Verification items for the finished model (mm, model axes). A direction names the side the tool comes from. Round coordinates to 2 decimals unless told otherwise and drop trailing zeros. Write each loop counter-clockwise with the first axis right and the second up, starting at its lowest first coordinate (ties: lowest second). Pieces come first, ordered by that corner, then holes.
from build123d import *

# Parameters (mm, degrees)
CYLINDER002_R          = 7
CYLINDER002_DEPTH      = 15
CYLINDER002_ROLL_ANGLE = -90
PAD_DEPTH              = 15
CYLINDER003_R          = 12
CYLINDER003_DEPTH      = 30
CYLINDER_R             = 11
CYLINDER_DEPTH         = 7
BOX_W                  = 30
BOX_H                  = 15
BOX_DEPTH              = 30
CYLINDER001_R          = 15
CYLINDER001_DEPTH      = 15
CYLINDER001_ROLL_ANGLE = -90
CYLINDER004_R          = 15
CYLINDER004_DEPTH      = 45


with BuildPart() as cylinder001:
    # Cylinder002 → Cylinder002 (new body)
    with BuildSketch(Plane.XY):
        Circle(CYLINDER002_R)
    extrude(amount=CYLINDER002_DEPTH)


with BuildPart() as cylinder001_1:
    # Cylinder002 roll: moved
    add(cylinder001.part.rotate(Axis((0, 0, 0), (1, 0, 0)), CYLINDER002_ROLL_ANGLE))


with BuildPart() as cylinder001_2:
    # Cylinder002 placement: moved
    add(cylinder001_1.part.moved(Location((0, -7.5, 0))))


with BuildPart() as body:
    # Sketch → Pad (new body)
    with BuildSketch(Plane.XZ):
        Polygon((-7, 0), (7, 0), (15, -8), (15, -30), (-15, -30), (-15, -8), align=None)
    extrude(amount=-PAD_DEPTH)


with BuildPart() as body_1:
    # Body placement: moved
    add(body.part.moved(Location((0, -7.5, 0))))


with BuildPart() as common:
    # Cylinder003 → Cylinder003 (new body)
    with BuildSketch(Plane.XY.offset(-30)):
        Circle(CYLINDER003_R)
    extrude(amount=CYLINDER003_DEPTH)

    # Common: intersect Body
    add(body_1.part, mode=Mode.INTERSECT)


with BuildPart() as negative_fusion:
    # Cylinder → Cylinder (new body)
    with BuildSketch(Plane(origin=(0, -3.5, 0), x_dir=(0, 0, -1), z_dir=(0, 1, 0))):
        Circle(CYLINDER_R)
    extrude(amount=CYLINDER_DEPTH)

    # Fusion: union Cylinder001, Common
    add(cylinder001_2.part)
    add(common.part)


with BuildPart() as cube:
    # Box → Box (new body)
    with BuildSketch(Plane(origin=(-15, -7.5, -30), x_dir=(1, 0, 0), z_dir=(0, 0, 1))):
        with Locations((15, 7.5)):
            Rectangle(BOX_W, BOX_H)
    extrude(amount=BOX_DEPTH)


with BuildPart() as cut:
    # Cylinder001 → Cylinder001 (new body)
    with BuildSketch(Plane.XY):
        Circle(CYLINDER001_R)
    extrude(amount=CYLINDER001_DEPTH)


with BuildPart() as cut_1:
    # Cylinder001 roll: moved
    add(cut.part.rotate(Axis((0, 0, 0), (1, 0, 0)), CYLINDER001_ROLL_ANGLE))


with BuildPart() as cut_2:
    # Cylinder001 placement: moved
    add(cut_1.part.moved(Location((0, -7.5, 0))))

    # Fusion001: union Cube
    add(cube.part)

    # Cut: cut Negative Fusion
    add(negative_fusion.part, mode=Mode.SUBTRACT)


with BuildPart() as common001:
    # Cylinder004 → Cylinder004 (new body)
    with BuildSketch(Plane.XY.offset(-30)):
        Circle(CYLINDER004_R)
    extrude(amount=CYLINDER004_DEPTH)

    # Common001: intersect Cut
    add(cut_2.part, mode=Mode.INTERSECT)


solid = common001.part
Q1. Sectioned sample at C-C (y = -0.75). Enter the section's corners in (x, z), plus the area to 3 significant figures.
Recorded:
outline: (-14.98, -30) - (-11.98, -30) - (-11.98, -4.98) - (-10.45, -3.45) arc R11 cw (long way) to (10.45, -3.45) - (11.98, -4.98) - (11.98, -30) - (14.98, -30) - (14.98, 0.75) arc R15 ccw to (-14.98, 0.75) - close
area: 354 mm2
Q2. Tool access check on faces 1 (the cylindrical face through (0, -6, 7)), 2 (the cylindrical face through (-12, 0, -16)), 3 (the cylindrical face through (0, 0, 11)). Record the directions out of +Z, -Z, +X, -X, +Y, -Y that give a thin tool (end or side, any length) a straight path to the whole face; none if there is none.
Recorded:
face 1: -Z, +Y, -Y
face 2: -Z
face 3: none
Q3. Sectioned sample at B-B (x = 0). Enter the section's corners in (y, z), plus the area to 3 significant figures.
Recorded:
outline: (-7.5, 7) - (-3.5, 7) - (-3.5, 11) - (3.5, 11) - (3.5, 7) - (7.5, 7) - (7.5, 15) - (-7.5, 15) - close
area: 92.0 mm2
Q4. Sectioned sample at A-A (z = -20.5). Enter the section's corners in (x, y).
Recorded:
outline: (-12.99, -7.5) - (-9.37, -7.5) arc R12 cw to (-9.37, 7.5) - (-12.99, 7.5) arc R15 ccw to start; (9.37, -7.5) - (12.99, -7.5) arc R15 ccw to (12.99, 7.5) - (9.37, 7.5) arc R12 cw to start
Q5. Sectioned sample at D-D (z = -1). Enter the section's corners in (x, y), plus the area to 3 significant figures.
Recorded:
outline: (-12.99, -7.5) - (-8, -7.5) - (-8, -3.5) - (-10.95, -3.5) - (-10.95, 3.5) - (-8, 3.5) - (-8, 7.5) - (-12.99, 7.5) arc R15 ccw to start; (8, -7.5) - (12.99, -7.5) arc R15 ccw to (12.99, 7.5) - (8, 7.5) - (8, 3.5) - (10.95, 3.5) - (10.95, -3.5) - (8, -3.5) - close
area: 149 mm2
Q6. Depth check by flat-ended pin: P1, Ø6, axis at x = -5.5, y = -5.5, coming from the -Z side; P2, Ø8, axis at y = 5.5, z = -10, coming from the +X side; P3, Ø1.5, axis at y = 3, z = -6.5, coming from the -X side. Enter the tip coordinate at first touch or a pass-through.
Recorded:
P1: stops at z = -1.5
P2: stops at x = 14.92
P3: stops at x = -14.83
Q7. Material ranges on line 1 along X through (y, z) = (0.75, 0); line 2 along X through (y, z) = (3.75, -13.5); line 3 along Z through (x, y) = (-11.75, 0.25), recorded low to high.
Recorded:
line 1: x = -14.98 to -11, 11 to 14.98
line 2: x = -14.52 to -11.4, 11.4 to 14.52
line 3: z = -4.75 to 9.32
Q8. Release check for a two-part mould opening along X. For faces 4 (the flat face through (-3, -3.5, 7)), 5 (the cylindrical face through (-15, 0, -12)), 6 (the cylindrical face through (0, 0, 15)) record: released by +X, released by -X, zero draft, split by the parting line, or undercut.
Recorded:
face 4: undercut
face 5: released by -X
face 6: split by the parting line
